```python
from build123d import *

# Parameters (mm, degrees)
SKETCH1_R           = 5.000000000000002
BOSS_EXTRUDE1_DEPTH = 13
CUT_EXTRUDE1_DEPTH  = 12.5
FILLET4_R           = 2
FILLET5_R           = 0.5
FILLET6_R           = 2


with BuildPart() as part:
    # Sketch1 → Boss-Extrude1 (new body)
    with BuildSketch(Plane(origin=(0, 0, 0), x_dir=(1, 0, 0), z_dir=(0, 1, 0))):
        with Locations(Location((0, 0, 0), (0, 0, 90))):
            Circle(SKETCH1_R)
    extrude(amount=BOSS_EXTRUDE1_DEPTH)

    # Insert → Cut-Extrude1 (cut)
    with BuildSketch(Plane.XZ):
        with BuildLine():
            Line((-1.9999999999999991, 2.872281323269015), (-1.9999999999999991, -2.872281323269015))
            ThreePointArc((-1.9999999999999991, -2.872281323269015), (3.5, 0), (-1.9999999999999991, 2.872281323269015))
        make_face()
    extrude(amount=-CUT_EXTRUDE1_DEPTH, mode=Mode.SUBTRACT)

    # Fillet4
    # the kernel refuses this fillet: 2 mm, written as the material it adds along each edge
    with BuildSketch(Plane(origin=(-1.1e-16, 12.5, 0), x_dir=(-0.9999950652018582, 0, -0.0031415874858792743), z_dir=(-0.0031415874858792743, 0, 0.9999950652018582))) as fillet4_piece_1:
        with BuildLine():
            CenterArc((3.5000000000000004 - FILLET4_R, FILLET4_R), FILLET4_R, 270, 90)
            Line((3.5000000000000004 - FILLET4_R, 0), (3.5000000000000004, 0))
            Line((3.5000000000000004, 0), (3.5000000000000004, FILLET4_R))
        make_face()
    revolve(axis=Axis((-1.1e-16, 12.5, 0), (0, -1, 0)), revolution_arc=359.64)
    with BuildSketch(Plane(origin=(-1.9999999999999991, 12.5, 7.872281323269015), x_dir=(0, -1, 0), z_dir=(0, 0, -1))) as fillet4_piece_2_section:
        with BuildLine():
            CenterArc((FILLET4_R, -FILLET4_R), FILLET4_R, 90, 90)
            Line((0, -FILLET4_R), (0, 0))
            Line((0, 0), (FILLET4_R, 0))
        make_face()
    fillet4_piece_2 = extrude(amount=15.74456264653803, mode=Mode.PRIVATE)
    fillet4_piece_2 = fillet4_piece_2 & Plane(origin=(-1.1e-16, 12.065491957530494, 0), x_dir=(-0.5714285714285712, 0, -0.8206518066482901), z_dir=(0, -1, 0)) * Cylinder(3.5, 40, mode=Mode.PRIVATE)
    add(fillet4_piece_2)

    # Fillet5
    fillet5_edges = [part.edges().sort_by_distance(p)[0] for p in [
        (3.5, 0, -4.4e-16),
        (-1.9999999999999991, 0, 0),
    ]]
    fillet(fillet5_edges, radius=FILLET5_R)

    # Fillet6
    fillet6_edges = [part.edges().sort_by_distance(p)[0] for p in [
        (-9.2e-16, 13, 5.000000000000002),
    ]]
    fillet(fillet6_edges, radius=FILLET6_R)


solid = part.part
```
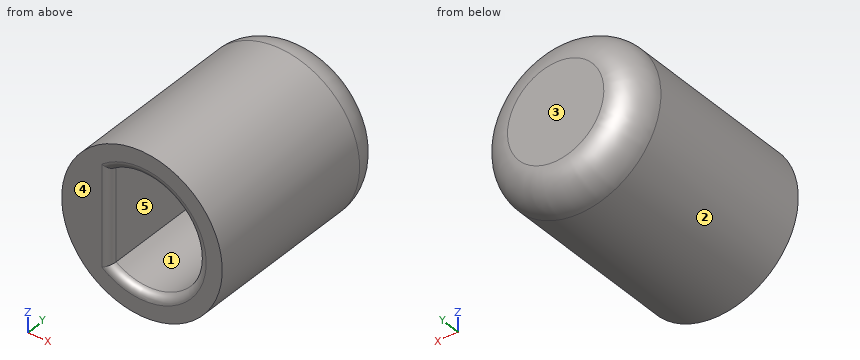
Can you work these out from the model? Positions are in its coordinate system, mm. Face numbers are marked on the shaded views. A direction names the side the tool comes from. Coordinates: 2 decimals unless noted, no trailing zeros. Loops run counter-clockwise (first coordinate to the right, second up) from the corner with the lowest first, then second, coordinate; pieces in that order, holes last. Notation, with made-up numbers: (82.25, 39.25) - (99.25, 39.25) arc R23 cw to (99.25, 76.25) - close; hole circle Ø11 at (-2.75, 33). An arc over 180 degrees is marked (long way). Answer as CSV lines item,"result". Start each with the question number.
1) Which directions (+Z, -Z, +X, -X, +Y, -Y) give clear straight access to the entire face, cutting with the end or side of a thin tool? Please do the marked faces 4 and 5.
2) For pin 1 (1 mm diameter, centred on y = 5.5, z = -2.5, fed in from -X); pin 2 (2 mm diameter, centred on y = 2.5, z = 4, fed in from -X); pin 3 (2 mm diameter, centred on x = 1, y = 11.5, fed in from -Z), each with a flat end and sliding along its axis, tell me the tip position at first contact or that it passes through.
3) Thinking about a two-plate mould opening in X: for the marked faces 1, 2 and 3, which applies, pulls with the +X half, pulls with the -X half, needs draft (parallel to the pull), parting line crosses it, or undercut?
4) Suppose I cut it at A-A (y = 10.25). Please give me the cut outline in (x, z).
5) I need wall thicknesses on line 1 (X direction, y = 6.75, z = 0); line 2 (X direction, y = 11, z = -0.25); line 3 (Z direction, x = 1.25, y = 0.75). Which ranges of each line are inside material? Lowest first, please. Write a range as from..to.
Check result:
1,face 4,"+Z, -Z, +X, -X, -Y"
1,face 5,"-Y"
2,pin 1,"stops at x = -4.58"
2,pin 2,"stops at x = -4"
2,pin 3,"stops at z = -5"
3,face 1,"undercut"
3,face 2,"parting line crosses it"
3,face 3,"needs draft"
4,outline,"circle Ø10 at (0, 0); hole (-2, -2.87) arc R3.5 ccw (long way) to (-2, 2.87) - close"
5,line 1,"x = -5..-2, 3.5..5"
5,line 2,"x = -4.99..-1.94, 3.43..4.99"
5,line 3,"z = -4.84..-3.27, 3.27..4.84"
